from build123d import *

# Parameters (mm, degrees)
F2_R     = 10
F3_DEPTH = 46.4
F6_R     = 16.1602540378
F7_W     = 76.2340277433
F7_H     = 67.4281166866
F8_DEPTH = 24.8


with BuildPart() as f1:
    # F0 (on Top) → F1 (revolve)
    with BuildSketch(Plane.XY):
        with BuildLine():
            Line((0, -20), (0, 20))
            ThreePointArc((0, 20), (-20, 0), (0, -20))
        make_face()
    revolve(axis=Axis((0, 0, 0), (0, -1, 0)))

    # F2 (on Top) → F3 (join)
    with BuildSketch(Plane.XY):
        Circle(F2_R)
    extrude(amount=F3_DEPTH)

    # F4 (on face) → F5 (revolve)
    with BuildSketch(Plane.XY.offset(46.4)):
        with BuildLine():
            Line((0, 10), (0, 15))
            ThreePointArc((0, 15), (-15, 0), (0, -15))
            Line((0, -15), (0, -10))
            ThreePointArc((0, -10), (-10, 0), (0, 10))
        make_face()
    revolve(axis=Axis((0, 0, 46.4), (0, -1, 0)))

    # F6
    f6_edges = [f1.edges().sort_by_distance(p)[0] for p in [
        (-10, 0, 35.21966),
        (-10, 0, 17.320508),
    ]]
    fillet(f6_edges, radius=F6_R)

    # F7 (on Front) → F8 (intersect, symmetric)
    with BuildSketch(Plane.XZ):
        with Locations((2.2643767297, 23.6501595937)):
            Rectangle(F7_W, F7_H)
    extrude(amount=F8_DEPTH, both=True, mode=Mode.INTERSECT)


solid = f1.part
Read the model definition and answer for the solid it produces. Units are mm, in the model's axes. Give positions to 0.01 mm unless a question says otherwise; leave off trailing zeros. Loops run counter-clockwise (first coordinate to the right, second up) from the corner with the lowest first, then second, coordinate; pieces in that order, holes last. Notation, with made-up numbers: (63, 21) -> (119, 21) arc R12 cw to (119, 43) -> close; hole circle Ø2 at (80, 83.5). An arc over 180 degrees is marked (long way). Use a Markdown table: item, result.
Q1. Find the intervals of material crossed by line 1 along X through (y, z) = (0, 27.5); line 2 along Z through (x, y) = (-2, 5.5); line 3 along X through (y, z) = (7, 18), in increasing order.
Solved:
| item | result |
|---|---|
| line 1 | x = -10 to 10 |
| line 2 | z = -10.06 to 46.4, 54.51 to 57.36 |
| line 3 | x = -9.22 to 9.22 |
Q2. Determine the mould class of faces 1 (the face through (9.54, 3, 27.19)), 2 (the face through (0, 0, 46.4)), 3 (the face through (0, 0, -10.064)) for opening direction X: pulls with the +X half, pulls with the -X half, needs draft (parallel to the pull), parting line crosses it, or undercut.
Solved:
| item | result |
|---|---|
| face 1 | parting line crosses it |
| face 2 | undercut |
| face 3 | needs draft |
Q3. Section C-C, the plane z = 43.5 is taken. Determine the outline of the cut face in (x, y), then the cut area to 3 significant figures.
Solved:
| item | result |
|---|---|
| outline | circle Ø29.43 at (0, 0) |
| area | 680 mm^2 |
Q4. Each of these flat-tipped pins is pushed along its axis until it touches: pin 1 (3 mm diameter, centred on y = 8, z = -10, fed in from +X); pin 2 (2 mm diameter, centred on y = 0.5, z = 22, fed in from -X); pin 3 (2 mm diameter, centred on x = -9, z = 17.5, fed in from -Y). Where does it stop, or does it pass through?
Solved:
| item | result |
|---|---|
| pin 1 | stops at x = 16.5 |
| pin 2 | stops at x = -10.49 |
| pin 3 | stops at y = -8.98 |
Q5. Section A-A, the plane z = 52 is taken. Determine the outline of the cut face in (x, y), then the cut area to 3 significant figures.
Solved:
| item | result |
|---|---|
| outline | circle Ø27.83 at (0, 0); hole circle Ø16.57 at (0, 0) |
| area | 393 mm^2 |
Q6. Section B-B, the plane z = -1.5 is taken. Determine the outline of the cut face in (x, y), then the cut area to 3 significant figures.
Solved:
| item | result |
|---|---|
| outline | circle Ø39.89 at (0, 0) |
| area | 1,250 mm^2 |
